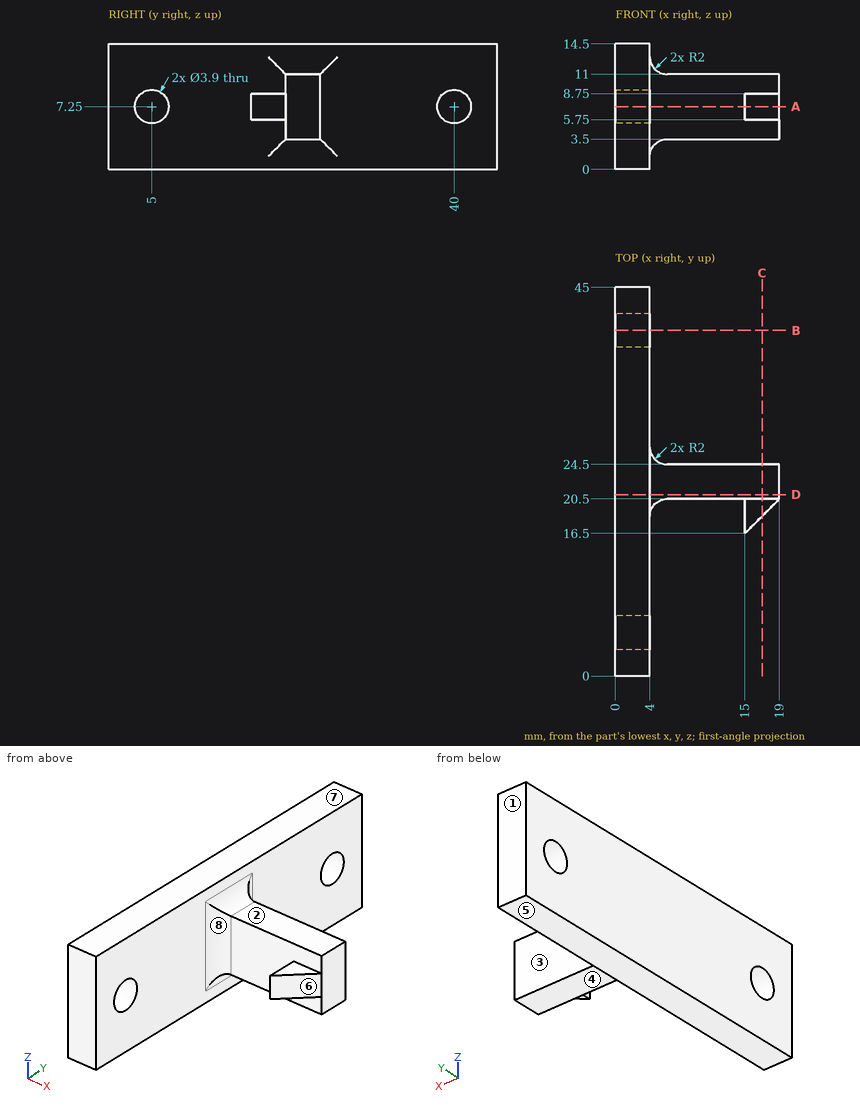
The figure shows three views and two pictorial views of one solid part (mm, origin at its lowest corner). Answer the questions. A direction names the side the tool comes from. Give positions to 0.01 mm unless a question says otherwise; leave off trailing zeros. Write each loop counter-clockwise with the first axis right and the second up, starting at its lowest first coordinate (ties: lowest second). Pieces come first, ordered by that corner, then holes. Notation, with made-up numbers: M 27,58 L 64,58 A22 ccw 64,81 Z; hole C 26,-9.75 d6. An arc over 180 degrees is marked long. One line per item, written item: value. Start each with the question number.
(1) Find section A-A (z = 7.25). Determine the outline of the cut face in (x, y), plus the area to 3 significant figures.
(2) Find section C-C (x = 17). Determine the outline of the cut face in (y, z), plus the area to 3 significant figures.
(3) A tool of negligible diameter and unlimited length cuts with its end or side. For the marked faces 1, 2, 3, 4 and 5, from which of +Z, -Z, +X, -X, +Y, -Y can it reach the whole face along a straight path? Write none if from no direction.
(4) Find section B-B (y = 40). Determine the outline of the cut face in (x, z), plus the area to 3 significant figures.
(5) Flat-ended cylindrical pins translate along their axes: pin 1 Ø2 at (x, y) = (18, 18.5) entering from -Z; pin 2 Ø3 at (x, z) = (7, 6.5) entering from +Y; pin 3 Ø4.5 at (y, z) = (40, 7.25) entering from +X. Find the tip coordinate at first contact, or state that the pin passes through.
(6) Determine the mould class of the marked faces 6, 7 and 8 for opening direction X: pulls with the +X half, pulls with the -X half, needs draft (parallel to the pull), parting line crosses it, or undercut.
(7) Find section D-D (y = 21). Determine the outline of the cut face in (x, z), plus the area to 3 significant figures.
(8) Find the intervals of material crossed by line 1 (Y direction, x = 2.6, z = 7.25); line 2 (Y direction, x = 3.5, z = 9); line 3 (Y direction, x = 16.75, z = 10.25), in increasing order.
Results below:
1. outline: M 0,0 L 4,0 L 4,3.05 L 0,3.05 Z; M 0,6.95 L 4,6.95 L 4,18.5 A2 cw 6,20.5 L 15,20.5 L 15,16.5 L 19,20.5 L 19,24.5 L 6,24.5 A2 cw 4,26.5 L 4,38.05 L 0,38.05 Z; M 0,41.95 L 4,41.95 L 4,45 L 0,45 Z
1. area: 219 mm^2
2. outline: M 18.5,5.75 L 20.5,5.75 L 20.5,3.5 L 24.5,3.5 L 24.5,11 L 20.5,11 L 20.5,8.75 L 18.5,8.75 Z
2. area: 36.0 mm^2
3. face 1: +Z, -Z, +X, -X, +Y
3. face 2: +Z, +X, +Y, -Y
3. face 3: +Z, -Z, +X, +Y
3. face 4: -Z, +X, +Y, -Y
3. face 5: -Z, +X, -X, +Y, -Y
4. outline: M 0,0 L 4,0 L 4,5.3 L 0,5.3 Z; M 0,9.2 L 4,9.2 L 4,14.5 L 0,14.5 Z
4. area: 42.4 mm^2
5. pin 1: stops at z = 5.75
5. pin 2: stops at y = 24.56
5. pin 3: stops at x = 4
6. face 6: pulls with the +X half
6. face 7: needs draft
6. face 8: undercut
7. outline: M 0,0 L 4,0 L 4,1.5 A2 cw 6,3.5 L 19,3.5 L 19,11 L 6,11 A2 cw 4,13 L 4,14.5 L 0,14.5 Z
7. area: 172 mm^2
8. line 1: y = 0 to 3.05, 6.95 to 38.05, 41.95 to 45
8. line 2: y = 0 to 4.14, 5.86 to 39.14, 40.86 to 45
8. line 3: y = 20.5 to 24.5
